Input: part model. Units: mm. Frame: model coordinates. Face numbers are marked on the shaded views. A direction names the side the tool comes from. Give positions to 0.01 mm unless a question says otherwise; leave off trailing zeros. Loops run counter-clockwise (first coordinate to the right, second up) from the corner with the lowest first, then second, coordinate; pieces in that order, holes last. Notation, with made-up numbers: M 17.5,-19.75 L 56.5,-19.75 A16 cw 56.5,-9.75 Z; hole C 73,32 d6. An arc over 180 degrees is marked long. Use a Markdown table: item, result. Add a question column.
from build123d import *

# Parameters (mm, degrees)
SKETCH1_W                = 57.9882
SKETCH1_H                = 17.70126
BOSS_EXTRUDE1_DEPTH      = 101.681600523
SKETCH5_W                = 15.24
SKETCH5_H                = 54.8132
CUT_EXTRUDE1_DEPTH       = 127
SKETCH6_R                = 4.49961
CUT_EXTRUDE2_DEPTH       = 127
CUT_EXTRUDE13_DEPTH      = 50.8
FILLET5_R                = 12.7
SKETCH14_R               = 3.96875
CUT_EXTRUDE14_DEPTH      = 88.9
CUT_EXTRUDE16_DEPTH      = 108.20606489
CUT_EXTRUDE16_DEPTH_BACK = 16.1925


with BuildPart() as part:
    # Sketch1 → Boss-Extrude1 (new body)
    with BuildSketch(Plane(origin=(0, 0, 0), x_dir=(0, 0, -1), z_dir=(1, 0, 0))):
        Rectangle(SKETCH1_W, SKETCH1_H)
    extrude(amount=BOSS_EXTRUDE1_DEPTH)

    # Sketch5 → Cut-Extrude1 (cut)
    with BuildSketch(Plane(origin=(0, 8.85063, 0), x_dir=(1, 0, 0), z_dir=(0, 1, 0))):
        with Locations((7.62, 0)):
            Rectangle(SKETCH5_W, SKETCH5_H)
    extrude(amount=-CUT_EXTRUDE1_DEPTH, mode=Mode.SUBTRACT)

    # Sketch6 → Cut-Extrude2 (cut)
    with BuildSketch(Plane(origin=(0, 8.85063, 0), x_dir=(1, 0, 0), z_dir=(0, 1, 0))):
        with BuildLine():
            ThreePointArc((15.24, 0), (16.557905256, 3.181704744), (19.73961, 4.49961))
            Line((19.73961, 4.49961), (15.24, 4.49961))
            Line((15.24, 4.49961), (15.24, 0))
        make_face()
        with Locations((19.73961, 0)):
            Circle(SKETCH6_R)
        with BuildLine():
            ThreePointArc((19.73961, -4.49961), (16.557905256, -3.181704744), (15.24, 0))
            Line((15.24, 0), (15.24, -4.49961))
            Line((15.24, -4.49961), (19.73961, -4.49961))
        make_face()
    extrude(amount=-CUT_EXTRUDE2_DEPTH, mode=Mode.SUBTRACT)

    # Sketch7 → Cut-Extrude13 (cut)
    with BuildSketch(Plane(origin=(101.681600523, 0, 0), x_dir=(0, 0, -1), z_dir=(1, 0, 0))):
        with BuildLine():
            Line((27.4066, 8.85063), (-27.4066, 8.85063))
            ThreePointArc((-27.4066, 8.85063), (0, -7.26313), (27.4066, 8.85063))
        make_face()
    extrude(amount=-CUT_EXTRUDE13_DEPTH, mode=Mode.SUBTRACT)

    # Fillet5
    fillet5_edges = [part.edges().sort_by_distance(p)[0] for p in [
        (50.881600523, 8.85063, 0),
    ]]
    fillet(fillet5_edges, radius=FILLET5_R)

    # Sketch14 → Cut-Extrude14 (cut)
    with BuildSketch(Plane(origin=(0, 0, -28.9941), x_dir=(-1, 0, 0), z_dir=(0, 0, -1))):
        with Locations(Location((-6.985, -0.89027, 0), (0, 0, 90))):
            Circle(SKETCH14_R)
    extrude(amount=-CUT_EXTRUDE14_DEPTH, mode=Mode.SUBTRACT)

    # Sketch18 → Cut-Extrude16 (cut, two sides: drawn at the far end of the back side and taken through both)
    with BuildSketch(Plane.XZ.offset(8.85063).offset(-CUT_EXTRUDE16_DEPTH_BACK)):
        with BuildLine():
            Line((38.18128, -27.4066), (38.18128, 27.4066))
            Line((38.18128, 27.4066), (15.24, 27.4066))
            Line((15.24, 27.4066), (15.24, 4.49961))
            Line((15.24, 4.49961), (19.73961, 4.49961))
            ThreePointArc((19.73961, 4.49961), (24.23922, 0), (19.73961, -4.49961))
            Line((19.73961, -4.49961), (15.24, -4.49961))
            Line((15.24, -4.49961), (15.24, -27.4066))
            Line((15.24, -27.4066), (38.18128, -27.4066))
        make_face()
    extrude(amount=CUT_EXTRUDE16_DEPTH + CUT_EXTRUDE16_DEPTH_BACK, mode=Mode.SUBTRACT)


solid = part.part
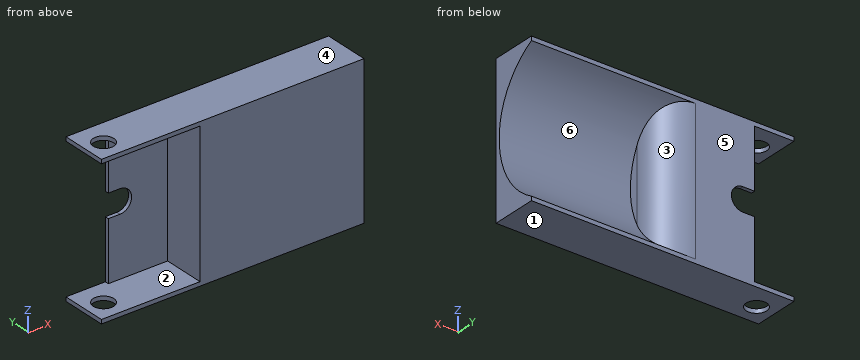
1) Reachability of the marked faces 1, 2 and 3 from +Z, -Z, +X, -X, +Y, -Y: full face, straight path, thin tool, end or side. Return the list, or none.
2) Contact query for flat-ended pins moving along their axis: P1, Ø25, axis at x = 25.5, z = -3, coming from the -Y side; P2, Ø10, axis at x = 86.5, z = -6.5, coming from the +Y side; P3, Ø0.8, axis at y = 8, z = -20.5, coming from the -X side; P4, Ø6.5, axis at x = 6.98, y = -0.89, coming from the +Z side. Output: stop coordinate, or through.
3) Section query A-A, the plane z = 0. Return the cut outline in (x, y), and give its area (3 significant figures).
4) Ray query, line 1 (Z direction, x = 27, y = 4.25); line 2 (Y direction, x = 25, z = -26); line 3 (Y direction, x = 51.5, z = 26.5). Return the intervals inside material, ascending. Write a range as [from, to].
5) Section query B-B, the plane y = -1.5. Return the cut outline in (x, z).
6) Section query D-D, the plane y = 5.25. Return the cut outline in (x, z).
7) Pull-direction query (Z, two-part tool) for the marked faces 4, 5 and 6; classes: pulls with the +Z half, pulls with the -Z half, needs draft (parallel to the pull), parting line crosses it, or undercut.
8) Section query C-C, the plane x = 53.5. Return the cut outline in (y, z), and give its area (3 significant figures).
Entries:
| question | item | result |
|---|---|---|
| 1 | face 1 | -Z, +X, -X, +Y, -Y |
| 1 | face 2 | -X, -Y |
| 1 | face 3 | +X, +Y |
| 2 | P1 | stops at y = 7.34 |
| 2 | P2 | stops at y = -5.08 |
| 2 | P3 | stops at x = 15.24 |
| 2 | P4 | passes through |
| 3 | outline | M 24.24,7.34 L 38.18,7.34 L 38.18,-8.85 L 101.68,-8.85 L 101.68,-7.26 L 50.88,-7.26 L 50.88,-3.85 A12.7 ccw 38.18,8.85 L 24.24,8.85 Z |
| 3 | area | 292 mm² |
| 4 | line 1 | z = [-28.99, -27.41], [27.41, 28.99] |
| 4 | line 2 | y = [7.34, 8.85] |
| 4 | line 3 | y = [-8.85, 7.32] |
| 5 | outline | M 0,-28.99 L 3.06,-28.99 L 3.06,-27.41 L 0,-27.41 Z; M 0,27.41 L 3.06,27.41 L 3.06,28.99 L 0,28.99 Z; M 10.91,-28.99 L 101.68,-28.99 L 101.68,-18.12 L 50.66,-18.12 L 50.66,18.12 L 101.68,18.12 L 101.68,28.99 L 10.91,28.99 L 10.91,27.41 L 38.18,27.41 L 38.18,-27.41 L 10.91,-27.41 Z |
| 6 | outline | M 0,-28.99 L 101.68,-28.99 L 101.68,-25.07 L 47.04,-25.07 L 47.04,25.07 L 101.68,25.07 L 101.68,28.99 L 0,28.99 L 0,27.41 L 38.18,27.41 L 38.18,-27.41 L 0,-27.41 Z |
| 7 | face 4 | pulls with the +Z half |
| 7 | face 5 | needs draft |
| 7 | face 6 | undercut |
| 8 | outline | M -8.85,-28.99 L 8.85,-28.99 L 8.85,-27.41 A31.36 cw 8.85,27.41 L 8.85,28.99 L -8.85,28.99 Z |
| 8 | area | 399 mm² |
